Build history of the part. All positions in model axes, mm. Face numbers are marked on the shaded views. A direction names the side the tool comes from. Give positions to 0.01 mm unless a question says otherwise; leave off trailing zeros. Write each loop counter-clockwise with the first axis right and the second up, starting at its lowest first coordinate (ties: lowest second). Pieces come first, ordered by that corner, then holes.
from build123d import *

# Parameters (mm, degrees)
F0_W     = 50.8
F0_H     = 4.2545
F0_H_2   = 23.241
F1_DEPTH = 4.7625
F2_DEPTH = 17.78
F4_DEPTH = 50.801


with BuildPart() as f1:
    # F0 (on Front) → F1 (new body)
    with BuildSketch(Plane.XZ):
        with Locations((0, 13.74775)):
            Rectangle(F0_W, F0_H)
        Rectangle(F0_W, F0_H_2)
        with Locations((0, -13.74775)):
            Rectangle(F0_W, F0_H)
    extrude(amount=-F1_DEPTH)

    # F0 (on Front) → F2 (join)
    with BuildSketch(Plane.XZ):
        with Locations((0, 13.74775)):
            Rectangle(F0_W, F0_H)
        with Locations((0, -13.74775)):
            Rectangle(F0_W, F0_H)
    extrude(amount=F2_DEPTH)

    # F3 (on face) → F4 (cut, through all)
    with BuildSketch(Plane(origin=(-25.4, 0, 0), x_dir=(0, -1, 0), z_dir=(-1, 0, 0))):
        with BuildLine():
            Line((0, 11.6205), (0.79375, 11.6205))
            ThreePointArc((0.79375, 11.6205), (-0.5612660076, 12.1817660076), (0, 10.82675))
            Line((0, 10.82675), (0, 11.6205))
        make_face()
        with BuildLine():
            Line((0, -11.6205), (0, -10.82675))
            ThreePointArc((0, -10.82675), (-0.5612660076, -12.1817660076), (0.79375, -11.6205))
            Line((0.79375, -11.6205), (0, -11.6205))
        make_face()
    extrude(amount=-F4_DEPTH, mode=Mode.SUBTRACT)


solid = f1.part
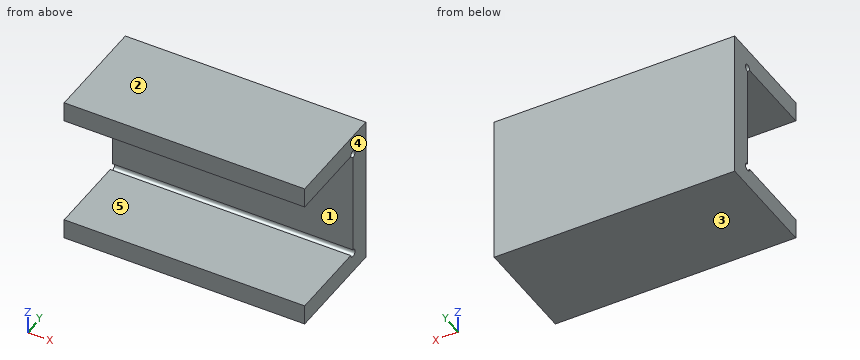
1. Drill centre lines: line 1 along Z through (x, y) = (-3, -12.75) (1 decimal); line 2 along Y through (x, z) = (-11.5, -7); line 3 along Y through (x, z) = (-3, 12). Where is each one in solid material? Low to high.
2. Saw through at A-A on y = -4.5. Give the cut face in (x, z) (1 decimal).
3. 3-axis set-ups, long thin cutter, end or side, ignore diameter. For the marked faces 4 and 5: which of +Z, -Z, +X, -X, +Y, -Y reach the whole face in a straight line?
4. Drop a flat-ended pin along its axis: pin 1 (6 mm diameter, centred on x = 7.5, z = 7.5, fed in from -Y). Give the stop position or say it passes through.
5. Mould opens along Z. For the marked faces 1, 2 and 3 say: pulls with the +Z half, pulls with the -Z half, needs draft (parallel to the pull), parting line crosses it, or undercut.
6. Saw through at B-B on x = -7. Give the cut face in (y, z) (1 decimal), plus the area to 3 significant figures.
7. Saw through at C-C on z = 2. Give the cut face in (x, y), plus the area to 3 significant figures.
Outcome:
1. line 1: z = -15.9 to -11.6, 11.6 to 15.9
1. line 2: y = 0 to 4.76
1. line 3: y = -17.78 to -0.7, 0.7 to 4.76
2. outline: (-25.4, -15.9) - (25.4, -15.9) - (25.4, -11.6) - (-25.4, -11.6) - close; (-25.4, 11.6) - (25.4, 11.6) - (25.4, 15.9) - (-25.4, 15.9) - close
3. face 4: +Z, -Z, +X, +Y, -Y
3. face 5: +X, -X, -Y
4. pin 1: stops at y = 0
5. face 1: undercut
5. face 2: pulls with the +Z half
5. face 3: pulls with the -Z half
6. outline: (-17.8, -15.9) - (4.8, -15.9) - (4.8, 15.9) - (-17.8, 15.9) - (-17.8, 11.6) - (-0.8, 11.6) arc R0.8 cw (long way) to (0, 10.8) - (0, -10.8) arc R0.8 cw (long way) to (-0.8, -11.6) - (-17.8, -11.6) - close
6. area: 300 mm2
7. outline: (-25.4, 0) - (25.4, 0) - (25.4, 4.76) - (-25.4, 4.76) - close
7. area: 242 mm2
